CAD build for the part. Positions are in the model's coordinates, mm. Face numbers are marked on the shaded views. Round coordinates to 2 decimals unless told otherwise and drop trailing zeros. Order: outer loops, then holes, each group sorted by start corner. A loop starts at its lowest first (then second) coordinate and runs counter-clockwise, first axis right, second up. Notation, with made-up numbers: (89, 65.5) - (103, 65.5) arc R29 cw to (103, 93.5) - close; hole circle Ø2 at (73, 85). An arc over 180 degrees is marked (long way). Write item = value, one per line.
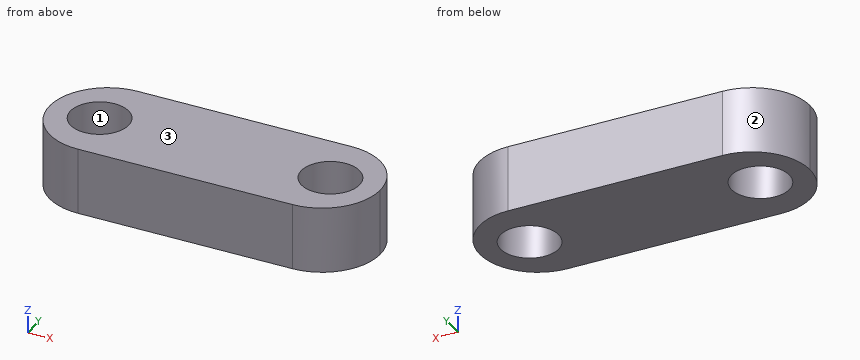
from build123d import *

# Parameters (mm, degrees)
SKETCH1_W           = 20
SKETCH1_H           = 7
SKETCH1_R           = 1.75
BOSS_EXTRUDE1_DEPTH = 4
FILLET1_R           = 3.5


with BuildPart() as part:
    # Sketch1 → Boss-Extrude1 (new body)
    with BuildSketch(Plane.XY):
        Rectangle(SKETCH1_W, SKETCH1_H)
        with Locations((-7, 0)):
            Circle(SKETCH1_R, mode=Mode.SUBTRACT)
        with Locations((7, 0)):
            Circle(SKETCH1_R, mode=Mode.SUBTRACT)
    extrude(amount=BOSS_EXTRUDE1_DEPTH)

    # Fillet1
    fillet1_edges = [part.edges().sort_by_distance(p)[0] for p in [
        (-10, 3.5, 2),
        (-10, -3.5, 2),
        (10, -3.5, 2),
        (10, 3.5, 2),
    ]]
    fillet(fillet1_edges, radius=FILLET1_R - 0.0001)  # a hair under: the kernel refuses the full size


solid = part.part
(1) Pull direction X, two halves, no side cores. Call the marked faces 1, 2 and 3: released by +X, released by -X, zero draft, split by the parting line, or undercut.
Solved:
face_1 = undercut
face_2 = released by -X
face_3 = zero draft
(2) Band-saw the part on D-D on y = -0.75. List the corners of the cut face in (x, z).
Solved:
outline = (-9.92, 0) - (-8.58, 0) - (-8.58, 4) - (-9.92, 4) - close; (-5.42, 0) - (5.42, 0) - (5.42, 4) - (-5.42, 4) - close; (8.58, 0) - (9.92, 0) - (9.92, 4) - (8.58, 4) - close
(3) Band-saw the part on B-B on y = 0.5. List the corners of the cut face in (x, z), plus the area to 3 significant figures.
Solved:
outline = (-9.96, 0) - (-8.68, 0) - (-8.68, 4) - (-9.96, 4) - close; (-5.32, 0) - (5.32, 0) - (5.32, 4) - (-5.32, 4) - close; (8.68, 0) - (9.96, 0) - (9.96, 4) - (8.68, 4) - close
area = 52.9 mm²
(4) Band-saw the part on A-A on x = -6. List the corners of the cut face in (y, z).
Solved:
outline = (-3.5, 0) - (-1.44, 0) - (-1.44, 4) - (-3.5, 4) - close; (1.44, 0) - (3.5, 0) - (3.5, 4) - (1.44, 4) - close
(5) Drop flat-ended pins along their axis: pin 1 (4 mm diameter, centred on x = 7, y = 0, fed in from +Z); pin 2 (1 mm diameter, centred on x = 7, y = 0, fed in from -Z); pin 3 (1 mm diameter, centred on y = -1, z = 1.5, fed in from -X). Give the stop position or say it passes through.
Solved:
pin_1 = 4
pin_2 = through
pin_3 = -9.96
(6) Probe line 1 along X through (y, z) = (0.75, 3.8); line 2 along Y through (x, z) = (7, 3.25); line 3 along Y through (x, z) = (-5.5, 2.9). List the from-to ranges inside material, lowest first.
Solved:
line_1 = -9.92 to -8.58, -5.42 to 5.42, 8.58 to 9.92
line_2 = -3.46 to -1.75, 1.75 to 3.46
line_3 = -3.5 to -0.9, 0.9 to 3.5
(7) Band-saw the part on C-C on z = 1.2. Count the separate pieces of the cut face and the enclosed holes in it, plus the area to 3 significant figures.
Solved:
separate_pieces = 1
enclosed_holes = 2
area = 110 mm²
